Input: part model. Units: mm. Frame: model coordinates. A direction names the side the tool comes from. Give positions to 0.01 mm unless a question says otherwise; leave off trailing zeros. Write each loop counter-clockwise with the first axis right and the second up, starting at its lowest first coordinate (ties: lowest second). Pieces come first, ordered by that corner, then holes. Notation, with made-up numbers: (65.5, 15) -> (92.5, 15) arc R19 ccw to (92.5, 41) -> close; hole circle Ø4 at (51, -20.75). An arc over 180 degrees is marked (long way). Return JSON: item names as keys, results as strings. Group by question number.
Item 1: Section C-C, the plane z = 881.5. Return loops of the section in (x, y).
Item 2: Line query: line 1 (Z direction, x = 472, y = -29); line 2 (X direction, y = -173, z = 506); line 3 (Y direction, x = 599.5, z = 1856). Output: solid intervals per line, ascending. Write a range as [from, to].
Item 3: Section D-D, the plane z = 1285. Return loops of the section in (x, y).
Item 4: Set-up query: faces 1 (the face through (19, -170, 482)), 2 (the face through (473, -180, 2244)), 3 (the face through (16, -336, 634)). Return all of +Z, -Z, +X, -X, +Y, -Y with unobstructed straight access to the full face (end or side cutting, diameter ignored); none if empty.
Item 5: Section A-A, the plane y = -125.5. Return loops of the section in (x, z).
Item 6: Section B-B, the plane x = 355. Return loops of the section in (y, z).
from build123d import *

# Parameters (mm, degrees)
F0_W      = 958
F0_H      = 2263
F1_DEPTH  = 336
F2_W      = 920
F2_H      = 856
F2_H_2    = 1290
F3_DEPTH  = 317
F3_FACE_W = 920
F3_FACE_H = 856
F4_DEPTH  = 25


with BuildPart() as f1:
    # F0 (on Front) → F1 (new body)
    with BuildSketch(Plane.XZ):
        with Locations((479, 1131.5)):
            Rectangle(F0_W, F0_H)
    extrude(amount=F1_DEPTH)

    # F2 (on face) → F3 (cut)
    with BuildSketch(Plane.XZ.offset(336)):
        with Locations((479, 488)):
            Rectangle(F2_W, F2_H)
        with Locations((479, 1599)):
            Rectangle(F2_W, F2_H_2)
    extrude(amount=-F3_DEPTH, mode=Mode.SUBTRACT)

    # F3_face (on face) → F4 (cut)
    with BuildSketch(Plane(origin=(479, -19, 488), x_dir=(1, 0, 0), z_dir=(0, -1, 0))):
        Rectangle(F3_FACE_W, F3_FACE_H)
    extrude(amount=-F4_DEPTH, mode=Mode.SUBTRACT)


solid = f1.part
Answer below:
{
 "1": {"outline": "(0, -336) -> (19, -336) -> (19, 0) -> (0, 0) -> close; (939, -336) -> (958, -336) -> (958, 0) -> (939, 0) -> close"},
 "2": {"line 1": "z = [0, 60], [916, 954], [2244, 2263]", "line 2": "x = [0, 19], [939, 958]", "line 3": "y = [-19, 0]"},
 "3": {"outline": "(0, -336) -> (19, -336) -> (19, -19) -> (939, -19) -> (939, -336) -> (958, -336) -> (958, 0) -> (0, 0) -> close"},
 "4": {"face 1": "+Y, -Y", "face 2": "-Y", "face 3": "+Z, -Z, +X, -X, -Y"},
 "5": {"outline": "(0, 0) -> (958, 0) -> (958, 2263) -> (0, 2263) -> close; hole (19, 60) -> (939, 60) -> (939, 916) -> (19, 916) -> close; hole (19, 954) -> (939, 954) -> (939, 2244) -> (19, 2244) -> close"},
 "6": {"outline": "(-336, 0) -> (0, 0) -> (0, 60) -> (-336, 60) -> close; (-336, 916) -> (0, 916) -> (0, 2263) -> (-336, 2263) -> (-336, 2244) -> (-19, 2244) -> (-19, 954) -> (-336, 954) -> close"}
}
